Can you work these out from the model? Positions are in its coordinate system, mm. A direction names the side the tool comes from. Coordinates: 2 decimals unless noted, no trailing zeros. Order: outer loops, then holes, each group sorted by start corner. A loop starts at its lowest first (then second) coordinate and runs counter-clockwise, first axis right, second up. Notation, with made-up numbers: (6, 74.25) -> (55, 74.25) arc R25 cw to (55, 111.25) -> close; hole circle Ø8 at (4.5, 87). An arc over 180 degrees is marked (long way). Return JSON: item names as keys, results as strings. Group by question number.
1) Thinking about a two-plate mould opening in X: for faces 5 (the flat face through (0, -6, 30)), 6 (the cylindrical face through (15.12, 4.76, 15.04)), 7 (the cylindrical face through (4.91, 1.55, 16.31)), which applies, +X half, -X half, draft (parallel to the pull), parting line (faces both ways), or undercut?
2) For pin 1 (1.5 mm diameter, centred on y = 7, z = 10.5, fed in from -X); pin 2 (2 mm diameter, centred on y = -7, z = 26, fed in from -X); pin 3 (3 mm diameter, centred on x = 4.5, y = 9, fed in from +Z), each with a flat end and sliding along its axis, tell me the tip position at first contact or that it passes through.
3) If I drill on probe 1 along Y at (x, z) = (0, 24); probe 2 along Y at (x, z) = (5, 18); probe 3 along X at (y, z) = (1.5, 8), over which ranges is the centre line in solid material (lowest first)? Write a range as from..to.
4) For faces 1 (the cylindrical face through (6.5, -1.462, 17.078)), 2 (the flat face through (0, 0, 0)), 3 (the cylindrical face through (7.53, -3.12, 16.69)), 4 (the cylindrical face through (-6.46, -1.46, 17.08)), which set-ups out of +Z, -Z, +X, -X, +Y, -Y let a thin tool reach every point of the face, with its end or its side?
5) If we section it at B-B, the plane x = 0: Please give me the cut outline in (y, z), then the cut area to 3 significant figures.
6) If we section it at A-A, the plane z = 11: Please give me the cut outline in (x, y).
from build123d import *

# Parameters (mm, degrees)
F0_R      = 15.85
F0_R_2    = 5.15
F1_DEPTH  = 30
F2_R      = 12.85
F2_R_2    = 8.15
F3_DEPTH  = 40
F4_R      = 12.65
F4_R_2    = 8.9
F5_DEPTH  = 40
F10_R     = 0.5
F11_R     = 15.35
F12_DEPTH = 3


# Not quite as in the source:
# - a feature names something its author has since deleted; it is built from what else it names


with BuildPart() as f1:
    # F0 (on Top) → F1 (new body)
    with BuildSketch(Plane.XY):
        Circle(F0_R)
        Circle(F0_R_2, mode=Mode.SUBTRACT)
    extrude(amount=F1_DEPTH)

    # F2 (on face) → F3 (cut)
    with BuildSketch(Plane.XY.offset(30)):
        Circle(F2_R)
        Circle(F2_R_2, mode=Mode.SUBTRACT)
    extrude(amount=-F3_DEPTH, mode=Mode.SUBTRACT)

    # F4 (on face) → F5 (cut)
    with BuildSketch(Plane(origin=(0, 0, 0), x_dir=(1, 0, 0), z_dir=(0, 0, -1))):
        Circle(F4_R)
        Circle(F4_R_2, mode=Mode.SUBTRACT)
    extrude(amount=-F5_DEPTH, mode=Mode.SUBTRACT)

    # F7 (on Right) → F9 (revolve, cut)
    with BuildSketch(Plane.YZ):
        with BuildLine():
            Line((1.4, 5), (1.4, 30))
            Line((1.4, 30), (0, 30))
            Line((0, 30), (-1.4, 30))
            Line((-1.4, 30), (-1.4, 5))
            ThreePointArc((-1.4, 5), (-0.9899494937, 4.0100505063), (0, 3.6))
            ThreePointArc((0, 3.6), (0.9899494937, 4.0100505063), (1.4, 5))
        make_face()
    revolve(axis=Axis((0, -340, 29.7196172178), (0, 0, 1)), mode=Mode.SUBTRACT)

    # F10
    f10_edges = [f1.edges().sort_by_distance(p)[0] for p in [
        (-14.307042, 1.100086, 30),
        (14.307042, 1.100086, 30),
        (6.50553, 1.338011, 30),
        (-6.50553, 1.338011, 30),
        (14.248226, -1.699914, 30),
        (-14.248226, -1.699914, 30),
        (-6.478795, -1.461989, 30),
        (6.478795, -1.461989, 30),
        (-15.85, 0, 0),
    ]]
    fillet(f10_edges, radius=F10_R)

    # F11 (on face) → F12 (join)
    with BuildSketch(Plane(origin=(0, 0, 0), x_dir=(1, 0, 0), z_dir=(0, 0, -1))):
        Circle(F11_R)
    extrude(amount=-F12_DEPTH)


solid = f1.part
Result sheet:
{
 "1": {"face 5": "draft", "face 6": "parting line", "face 7": "undercut"},
 "2": {"pin 1": "stops at x = -14.57", "pin 2": "stops at x = -14.67", "pin 3": "stops at z = 3"},
 "3": {"probe 1": "y = -15.85..-12.85, -8.15..-5.15, 5.15..8.15, 12.85..15.85", "probe 2": "y = -15.04..-11.84, -6.44..-1.44, 1.36..6.44, 11.84..15.04", "probe 3": "x = -15.78..-12.76, -8.01..-4.93, 4.93..8.01, 12.76..15.78"},
 "4": {"face 1": "+Z, +X", "face 2": "-Z, +X, -X, +Y, -Y", "face 3": "+Z", "face 4": "+Z, -X"},
 "5": {"outline": "(-15.85, 0.5) arc R0.5 ccw to (-15.35, 0) -> (15.35, 0) arc R0.5 ccw to (15.85, 0.5) -> (15.85, 30) -> (12.85, 30) -> (12.85, 3) -> (8.15, 3) -> (8.15, 30) -> (5.15, 30) -> (5.15, 3) -> (-5.15, 3) -> (-5.15, 30) -> (-8.15, 30) -> (-8.15, 3) -> (-12.85, 3) -> (-12.85, 30) -> (-15.85, 30) -> close", "area": "419 mm2"},
 "6": {"outline": "(-15.82, 1.03) arc R341.4 cw to (-12.8, 1.16) arc R12.85 cw to (12.8, 1.16) arc R341.4 cw to (15.82, 1.03) arc R15.85 ccw to start; (-15.75, -1.77) arc R15.85 ccw to (15.75, -1.77) arc R338.6 ccw to (12.74, -1.64) arc R12.85 cw to (-12.74, -1.64) arc R338.6 ccw to start; (-8.04, 1.31) arc R341.4 cw to (-4.97, 1.36) arc R5.15 cw to (4.97, 1.36) arc R341.4 cw to (8.04, 1.31) arc R8.15 ccw to start; (-8.01, -1.49) arc R8.15 ccw to (8.01, -1.49) arc R338.6 ccw to (4.95, -1.44) arc R5.15 cw to (-4.95, -1.44) arc R338.6 ccw to start"}
}
